```python
from build123d import *

# Parameters (mm, degrees)
SKETCH1_W           = 4
SKETCH1_H           = 80.5
BOSS_EXTRUDE1_DEPTH = 71
BOSS_EXTRUDE2_START = -4
BOSS_EXTRUDE2_DEPTH = 4
BOSS_EXTRUDE3_DEPTH = 34.2
CUT_EXTRUDE1_DEPTH  = 13
CUT_EXTRUDE2_DEPTH  = 13
SKETCH6_R           = 1.7
CUT_EXTRUDE3_DEPTH  = 13
SKETCH7_R           = 3.25
CUT_EXTRUDE4_DEPTH  = 2.5
BOSS_EXTRUDE4_DEPTH = 44.5
SKETCH10_W          = 46.002383675
SKETCH10_H          = 61.711229379
CUT_EXTRUDE5_DEPTH  = 42
BOSS_EXTRUDE5_DEPTH = 4
CUT_EXTRUDE6_DEPTH  = 10.6
CUT_EXTRUDE7_REACH  = 148.85
SKETCH13_R          = 1.9
SKETCH14_W          = 25
SKETCH14_H          = 33.9
BOSS_EXTRUDE6_DEPTH = 1
CUT_EXTRUDE8_DEPTH  = 15
SKETCH16_W          = 10.4
SKETCH16_H          = 1.3
CUT_EXTRUDE9_DEPTH  = 15
BOSS_EXTRUDE7_DEPTH = 15
SKETCH19_W          = 33
SKETCH19_H          = 37.9
CUT_EXTRUDE10_DEPTH = 1
FILLET1_R           = 2


with BuildPart() as part:
    # Sketch1 → Boss-Extrude1 (new body)
    with BuildSketch(Plane.XY):
        with Locations((2, 40.25)):
            Rectangle(SKETCH1_W, SKETCH1_H)
        with BuildLine():
            Line((0, 80.5), (4, 80.5))
            ThreePointArc((4, 80.5), (16.5, 93), (29, 80.5))
            Line((29, 80.5), (33, 80.5))
            ThreePointArc((33, 80.5), (16.5, 97), (0, 80.5))
        make_face()
        with Locations((31, 40.25)):
            Rectangle(SKETCH1_W, SKETCH1_H)
    extrude(amount=BOSS_EXTRUDE1_DEPTH)

    # Sketch2 → Boss-Extrude2 (add)
    with BuildSketch(Plane.XY.offset(71).offset(BOSS_EXTRUDE2_START)):
        with BuildLine():
            Line((33, 48.5), (0, 48.5))
            Line((0, 48.5), (0, 80.5))
            ThreePointArc((0, 80.5), (16.5, 97), (33, 80.5))
            Line((33, 80.5), (33, 48.5))
        make_face()
    extrude(amount=BOSS_EXTRUDE2_DEPTH)

    # Sketch3 → Boss-Extrude3 (add)
    with BuildSketch(Plane(origin=(0, 0, 67), x_dir=(-1, 0, 0), z_dir=(0, 0, -1))):
        Polygon((-33, 0), (-33, 48.5), (-29, 48.5), (-4, 48.5), (0, 48.5), (0, 0), (-3.837905566, 0), (-4, 44.5), (-29, 44.5), (-29.162094434, 0), align=None)
    extrude(amount=-BOSS_EXTRUDE3_DEPTH)

    # Sketch4 → Cut-Extrude1 (cut)
    with BuildSketch(Plane(origin=(0, 0, 0), x_dir=(-1, 0, 0), z_dir=(0, 0, -1))):
        with BuildLine():
            Line((-4, 80.5), (-4, 0))
            Line((-4, 0), (0, 0))
            Line((0, 0), (0, 80.5))
            ThreePointArc((0, 80.5), (-16.5, 97), (-33, 80.5))
            Line((-33, 80.5), (-33, 0))
            Line((-33, 0), (-29, 0))
            Line((-29, 0), (-29, 80.5))
            ThreePointArc((-29, 80.5), (-16.5, 93), (-4, 80.5))
        make_face()
    extrude(amount=-CUT_EXTRUDE1_DEPTH, mode=Mode.SUBTRACT)

    # Sketch5 → Cut-Extrude2 (cut)
    with BuildSketch(Plane.XY.offset(71)):
        with BuildLine():
            ThreePointArc((26.5, 80.5), (16.5, 90.5), (6.5, 80.5))
            Line((6.5, 80.5), (26.5, 80.5))
        make_face()
        with BuildLine():
            Line((26.5, 80.5), (6.5, 80.5))
            ThreePointArc((6.5, 80.5), (16.5, 70.5), (26.5, 80.5))
        make_face()
    extrude(amount=-CUT_EXTRUDE2_DEPTH, mode=Mode.SUBTRACT)

    # Sketch6 → Cut-Extrude3 (cut)
    with BuildSketch(Plane.XY.offset(71)):
        with Locations((6.5, 70.5)):
            Circle(SKETCH6_R)
        with BuildLine():
            ThreePointArc((28.2, 70.5), (26.5, 72.2), (24.8, 70.5))
            Line((24.8, 70.5), (28.2, 70.5))
        make_face()
        with BuildLine():
            Line((28.2, 70.5), (24.8, 70.5))
            ThreePointArc((24.8, 70.5), (26.5, 68.8), (28.2, 70.5))
        make_face()
    extrude(amount=-CUT_EXTRUDE3_DEPTH, mode=Mode.SUBTRACT)

    # Sketch7 → Cut-Extrude4 (cut)
    with BuildSketch(Plane.XY.offset(71)):
        with Locations((6.5, 70.5)):
            Circle(SKETCH7_R)
        with Locations((26.5, 70.5)):
            Circle(SKETCH7_R)
    extrude(amount=-CUT_EXTRUDE4_DEPTH, mode=Mode.SUBTRACT)

    # Sketch9 → Boss-Extrude4 (add)
    with BuildSketch(Plane.XZ):
        Polygon((29.162094434, 101.2), (29.162094434, 71), (29, 71), (29, 120), align=None)
        Polygon((4, 120), (3.837905566, 101.2), (3.837905566, 71), (4, 71), align=None)
    extrude(amount=-BOSS_EXTRUDE4_DEPTH)

    # Sketch10 → Cut-Extrude5 (cut)
    with BuildSketch(Plane.XY.offset(101.2)):
        with Locations((17.24268837, 24.291112106)):
            Rectangle(SKETCH10_W, SKETCH10_H)
    extrude(amount=CUT_EXTRUDE5_DEPTH, mode=Mode.SUBTRACT)

    # Sketch11 → Boss-Extrude5 (add)
    with BuildSketch(Plane.XY.offset(101.2)):
        Polygon((29, 0), (4, 0), (0, 0), (0, 48.5), (33, 48.5), (33, 0), align=None)
    extrude(amount=BOSS_EXTRUDE5_DEPTH)

    # Sketch12 → Cut-Extrude6 (cut)
    with BuildSketch(Plane.XZ):
        Polygon((4, 13), (4, 101.2), (29, 101.2), (29, 13), (33, 13), (33, 105.2), (0, 105.2), (0, 13), align=None)
    extrude(amount=-CUT_EXTRUDE6_DEPTH, mode=Mode.SUBTRACT)

    # Cut-Extrude7: up to this face of the body (flat: up to its plane)
    cut_extrude7_end = Plane(part.part.faces().sort_by_distance((33, 41.673849147, 53.168159645))[0])
    # Sketch13 → Cut-Extrude7 (cut, up to the picked face)
    with BuildSketch(Plane.ZY, mode=Mode.PRIVATE) as cut_extrude7_sk1:
        with Locations((40.2, 38.3)):
            Circle(SKETCH13_R)
    cut_extrude7_tool1 = split(extrude(cut_extrude7_sk1.sketch, amount=-CUT_EXTRUDE7_REACH, mode=Mode.PRIVATE), bisect_by=cut_extrude7_end, keep=Keep.BOTH, mode=Mode.PRIVATE)
    # Sketch13 → Cut-Extrude7 (cut, up to the picked face)
    with BuildSketch(Plane.ZY, mode=Mode.PRIVATE) as cut_extrude7_sk2:
        with Locations((24.2, 38.3)):
            Circle(SKETCH13_R)
    cut_extrude7_tool2 = split(extrude(cut_extrude7_sk2.sketch, amount=-CUT_EXTRUDE7_REACH, mode=Mode.PRIVATE), bisect_by=cut_extrude7_end, keep=Keep.BOTH, mode=Mode.PRIVATE)
    add(cut_extrude7_tool1.solids().sort_by(Axis((0, 38.3, 40.2), (1, 0, 0)))[0], mode=Mode.SUBTRACT)
    add(cut_extrude7_tool2.solids().sort_by(Axis((0, 38.3, 24.2), (1, 0, 0)))[0], mode=Mode.SUBTRACT)

    # Sketch14 → Boss-Extrude6 (add)
    with BuildSketch(Plane(origin=(0, 0, 101.2), x_dir=(-1, 0, 0), z_dir=(0, 0, -1))):
        with Locations((-16.5, 27.55)):
            Rectangle(SKETCH14_W, SKETCH14_H)
    extrude(amount=BOSS_EXTRUDE6_DEPTH)

    # Sketch15 → Cut-Extrude8 (cut)
    with BuildSketch(Plane.XZ.offset(-10.6)):
        Polygon((26.7, 103.9), (6.3, 103.9), (6.3, 101.5), (16.5, 101.5), (26.7, 101.5), align=None)
    extrude(amount=-CUT_EXTRUDE8_DEPTH, mode=Mode.SUBTRACT)

    # Sketch16 → Cut-Extrude9 (cut)
    with BuildSketch(Plane.XZ.offset(-10.6)):
        with Locations((16.5, 104.55)):
            Rectangle(SKETCH16_W, SKETCH16_H)
    extrude(amount=-CUT_EXTRUDE9_DEPTH, mode=Mode.SUBTRACT)

    # Sketch17 → Boss-Extrude7 (add)
    with BuildSketch(Plane.XZ.offset(-25.6)):
        Polygon((26.7, 103.9), (21.7, 103.9), (21.7, 105.2), (11.3, 105.2), (11.3, 103.9), (6.3, 103.9), (6.3, 101.5), (26.7, 101.5), align=None)
    extrude(amount=BOSS_EXTRUDE7_DEPTH)

    # Sketch19 → Cut-Extrude10 (cut)
    with BuildSketch(Plane.XY.offset(105.2)):
        with Locations((16.5, 29.55)):
            Rectangle(SKETCH19_W, SKETCH19_H)
    extrude(amount=-CUT_EXTRUDE10_DEPTH, mode=Mode.SUBTRACT)

    # Fillet1
    fillet1_edges = [part.edges().sort_by_distance(p)[0] for p in [
        (16.5, 48.5, 104.2),
    ]]
    fillet(fillet1_edges, radius=FILLET1_R)


solid = part.part
```
Geometry check sheet. Reference: the model listing, model coordinates, mm. A direction names the side the tool comes from. Give positions to 0.01 mm unless a question says otherwise; leave off trailing zeros. Write each loop counter-clockwise with the first axis right and the second up, starting at its lowest first coordinate (ties: lowest second). Pieces come first, ordered by that corner, then holes.
1) Material ranges on L1, parallel to X at y = 37.5, z = 60; L2, parallel to X at y = 80.5, z = 69.7; L3, parallel to Z at x = 2.5, y = 74, recorded low to high.
2) Access from +Z, -Z, +X, -X, +Y, -Y to the whole of each face (thin tool, end or side, straight path). Record for faces 1 (the flat face through (16, 48.5, 86)), 2 (the flat face through (28, 69, 68.5)), 3 (the cylindrical face through (24.88, 69.99, 67.76)), 4 (the flat face through (16, 64, 67)).
3) Gauge pin test, flat ends, axial feed: pin 1 (2 mm diameter, centred on y = 64, z = 53, fed in from -X); pin 2 (1 mm diameter, centred on x = 20.5, y = 49.5, fed in from -Z); pin 3 (7.5 mm diameter, centred on x = 19.5, z = 77.5, fed in from -Y); pin 4 (4 mm diameter, centred on x = 26.5, y = 70.5, fed in from +Z). Record the tip position at first contact, or that the pin passes through.
4) Section check C-C, the plane z = 40.2. Record the boundary of the cut face in (x, y).
5) Section check D-D, the plane z = 74. Record the boundary of the cut face in (x, y), and give its area (3 significant figures).
6) Section check A-A, the plane y = 38.3. Record the boundary of the cut face in (x, z), and give its area (3 significant figures).
7) Release check for a two-part mould opening along Y. For faces 5 (the flat face through (16, 44.5, 83)), 6 (the flat face through (4, 45, 46)), 7 (the cylindrical face through (5.795, 67.327, 69.768)) record: pulls with the +Y half, pulls with the -Y half, needs draft (parallel to the pull), parting line crosses it, or undercut.
8) Section check B-B, the plane x = 16.5. Record the boundary of the cut face in (y, z).
Computed:
1. L1: x = 0 to 4, 29 to 33
1. L2: x = 0 to 6.5, 26.5 to 33
1. L3: z = 13 to 71
2. face 1: +Z, +X, -X, +Y
2. face 2: +Z
2. face 3: +Z, -Z
2. face 4: -Z, -Y
3. pin 1: stops at x = 0
3. pin 2: stops at z = 67
3. pin 3: stops at y = 44.5
3. pin 4: stops at z = 68.5
4. outline: (0, 10.6) - (4, 10.6) - (4, 36.4) - (0, 36.4) - close; (0, 40.2) - (4, 40.2) - (4, 80.5) arc R12.5 cw to (29, 80.5) - (29, 40.2) - (33, 40.2) - (33, 80.5) arc R16.5 ccw to (0, 80.5) - close; (29, 10.6) - (33, 10.6) - (33, 36.4) - (29, 36.4) - close
5. outline: (0, 10.6) - (4, 10.6) - (4, 44.5) - (29, 44.5) - (29, 10.6) - (33, 10.6) - (33, 48.5) - (0, 48.5) - close
5. area: 403 mm2
6. outline: (0, 13) - (4, 13) - (4, 22.3) - (0, 22.3) - close; (0, 26.1) - (4, 26.1) - (4, 38.3) - (0, 38.3) - close; (0, 42.1) - (4, 42.1) - (4, 100.2) - (29, 100.2) - (29, 42.1) - (33, 42.1) - (33, 104.2) - (0, 104.2) - close; (29, 13) - (33, 13) - (33, 22.3) - (29, 22.3) - close; (29, 26.1) - (33, 26.1) - (33, 38.3) - (29, 38.3) - close
6. area: 769 mm2
7. face 5: pulls with the -Y half
7. face 6: needs draft
7. face 7: undercut
8. outline: (10.6, 100.2) - (44.5, 100.2) - (44.5, 67) - (70.5, 67) - (70.5, 71) - (48.5, 71) - (48.5, 102.2) arc R2 ccw to (46.5, 104.2) - (10.6, 104.2) - close; (90.5, 67) - (93, 67) - (93, 13) - (97, 13) - (97, 71) - (90.5, 71) - close
